from build123d import *

# Parameters (mm, degrees)
F0_R     = 41.91
F0_R_2   = 39.624
F1_DEPTH = 12.7
F2_R     = 45.609327
F4_DEPTH = 1.905
F3_R     = 3.96875
F5_DEPTH = 25.4
F7_DEPTH = 5.334


with BuildPart() as f1:
    # F0 (on Top) → F1 (new body)
    with BuildSketch(Plane.XY):
        Circle(F0_R)
        Circle(F0_R_2, mode=Mode.SUBTRACT)
    extrude(amount=F1_DEPTH)

    # F2 (on Top) → F4 (join)
    with BuildSketch(Plane.XY):
        Circle(F2_R)
    extrude(amount=-F4_DEPTH)

    # F3 (on Top) → F5 (cut)
    with BuildSketch(Plane.XY):
        Circle(F3_R)
    extrude(amount=-F5_DEPTH, mode=Mode.SUBTRACT)

    # F6 (on Top) → F7 (cut)
    with BuildSketch(Plane.XY):
        Polygon((-5.480623, 2.9152), (-4.250295, 5.673185), (-26.960552, 25.830237), (-36.436632, 7.79836), align=None)
    extrude(amount=-F7_DEPTH, mode=Mode.SUBTRACT)


solid = f1.part
Build history of the part. All positions in model axes, mm. A direction names the side the tool comes from. Round coordinates to 2 decimals unless told otherwise and drop trailing zeros. Write each loop counter-clockwise with the first axis right and the second up, starting at its lowest first coordinate (ties: lowest second). Pieces come first, ordered by that corner, then holes. Notation, with made-up numbers: M 10,63 L 51,63 A30 cw 51,87 Z; hole C 21,12.5 d5. An arc over 180 degrees is marked long. Answer as a JSON object with one key per item and string values. Group by question number.
(1) Cut at D-D (x = 19). Give the cut face in (y, z) (3 decimals), and give its area (3 significant figures).
(2) Cut at C-C (z = 10). Give the cut face in (x, y), and give its area (3 significant figures).
(3) Flat gauge pins, fed straight in: pin 1 (8 mm diameter, centred on x = 18, y = -21, fed in from +Z); pin 2 (6 mm diameter, centred on x = -19, z = 8.5, fed in from -Y); pin 3 (8 mm diameter, centred on x = -6, z = 2.5, fed in from +Y); pin 4 (10.5 mm diameter, centred on x = 0, y = 0, fed in from -Z) (3 decimals). Where does each tip first touch, or does it go through?
(4) Mould opens along X. For faces 1 (the flat face through (-15.446, 15.611, -0.939)), 2 (the cylindrical face through (-9.887, -44.525, -0.939)), 3 (the flat face through (9, 1, -1.905)) say: pulls with the +X half, pulls with the -X half, needs draft (parallel to the pull), parting line crosses it, or undercut.
(5) Drill centre lines: L1, parallel to Y at x = 0, z = 3.75; L2, parallel to Y at x = 0, z = -0.8; L3, parallel to Z at x = 1, y = -21 (3 decimals). Where is each one in solid material? Low to high.
(6) Cut at A-A (y = 0). Give the cut face in (x, z) (3 decimals).
(7) Which spindle directions (+Z, -Z, +X, -X, +Y, -Y) get a long thin tool onto all of the face, cutting with end or side? Do faces 4 (the flat face through (8, 1, 0)), 5 (the flat face through (-31.632, 16.941, -0.939)), 6 (the flat face through (31, 25, 12.7)). Say none if no direction does.
Responses:
{
 "1": {"outline": "M -41.463,-1.905 L 41.463,-1.905 L 41.463,0 L 37.356,0 L 37.356,12.7 L 34.772,12.7 L 34.772,0 L -34.772,0 L -34.772,12.7 L -37.356,12.7 L -37.356,0 L -41.463,0 Z", "area": "224 mm2"},
 "2": {"outline": "C 0,0 d83.82; hole C 0,0 d79.25", "area": "586 mm2"},
 "3": {"pin 1": "stops at z = 0", "pin 2": "stops at y = -38.74", "pin 3": "stops at y = 45.52", "pin 4": "stops at z = -1.905"},
 "4": {"face 1": "undercut", "face 2": "parting line crosses it", "face 3": "needs draft"},
 "5": {"L1": "y = -41.91 to -39.62, 39.62 to 41.91", "L2": "y = -45.61 to -3.97, 3.97 to 45.61", "L3": "z = -1.905 to 0"},
 "6": {"outline": "M -45.609,-1.905 L -3.969,-1.905 L -3.969,0 L -39.624,0 L -39.624,12.7 L -41.91,12.7 L -41.91,0 L -45.609,0 Z; M 3.969,-1.905 L 45.609,-1.905 L 45.609,0 L 41.91,0 L 41.91,12.7 L 39.624,12.7 L 39.624,0 L 3.969,0 Z"},
 "7": {"face 4": "+Z", "face 5": "+Z, -Z", "face 6": "+Z, +X, -X, +Y, -Y"}
}
